For this review, take the finished solid that the model builds, in its own axes (mm). Coordinates: 2 decimals unless noted, no trailing zeros. Order: outer loops, then holes, each group sorted by start corner. A loop starts at its lowest first (then second) coordinate and runs counter-clockwise, first axis right, second up. Notation, with made-up numbers: (57, 3.25) -> (107, 3.25) arc R24 ccw to (107, 42.25) -> close; hole circle Ø7 at (62.25, 26). An arc over 180 degrees is marked (long way). Write item = value, one per line. Start each with the question number.
1) Consider section C-C on x = 88.9. Give the boundary of the cut face in (y, z).
2) Consider section B-B on z = -60.5. Give the boundary of the cut face in (x, y), and give its area (3 significant figures).
3) Consider section A-A on x = 50.8. Give the boundary of the cut face in (y, z), and give its area (3 significant figures).
4) Wall thickness on probe 1 along Z at (x, y) = (12.7, 3.75); probe 2 along X at (y, z) = (1.75, -31); probe 3 along X at (y, z) = (5, -19.05): over which ranges is each line inside the solid? List them lowest first. Write a range as [from, to].
5) Insertion check: pin 1 Ø6 at (x, z) = (50.8, -31.115) entering from -Y. The pin has a flat end and moves straight along its axis. Give the tip position at first contact, or say it passes through.
6) Consider section D-D on y = 4.5. State how many separate pieces and enclosed holes the cut face has, and give its area (3 significant figures).
7) Draft analysis for pull direction X (two halves, no side actions). For faces 1 (the face through (10.46, 3.13, -19.76)), 2 (the face through (101.6, 3, -35)), 3 (the face through (50, 3, -71.12)), 4 (the face through (0, 3, -35)), state which applies: +X half, -X half, draft (parallel to the pull), parting line (faces both ways), or undercut.
from build123d import *

# Parameters (mm, degrees)
SKETCH1_W                       = 101.6
SKETCH1_H                       = 71.12
BASE_DEPTH                      = 6.35
WOODSCREW_CLEARANCE_HOLES_D     = 4.699
WOODSCREW_CLEARANCE_HOLES_DEPTH = 6.35
WOODSCREW_CLEARANCE_HOLES_TIP   = 1.411722024
SHAFT_CLEARANCE_HOLE_D          = 10.2616
SHAFT_CLEARANCE_HOLE_DEPTH      = 6.35
SHAFT_CLEARANCE_HOLE_TIP        = 3.082895664
M5X0_8_TAPPED_HOLE1_D           = 4.2


with BuildPart() as part:
    # Sketch1 → base (new body)
    with BuildSketch(Plane(origin=(0, 0, 0), x_dir=(1, 0, 0), z_dir=(0, 1, 0))):
        with Locations((50.8, 35.56)):
            Rectangle(SKETCH1_W, SKETCH1_H)
    extrude(amount=BASE_DEPTH)

    # woodscrew clearance holes
    with Locations(Plane(origin=(0, 6.35, 0), x_dir=(1, 0, 0), z_dir=(0, 1, 0))):
        with Locations((12.7, 61.595), (88.9, 61.595), (88.9, 19.05), (12.7, 19.05)):
            Hole(WOODSCREW_CLEARANCE_HOLES_D / 2, depth=WOODSCREW_CLEARANCE_HOLES_DEPTH)
            with Locations((0, 0, -(WOODSCREW_CLEARANCE_HOLES_DEPTH + WOODSCREW_CLEARANCE_HOLES_TIP / 2))):  # 118° drill point
                Cone(0, WOODSCREW_CLEARANCE_HOLES_D / 2, WOODSCREW_CLEARANCE_HOLES_TIP, mode=Mode.SUBTRACT)

    # shaft clearance hole
    with Locations(Plane(origin=(0, 6.35, 0), x_dir=(1, 0, 0), z_dir=(0, 1, 0))):
        with Locations((50.8, 31.115)):
            Hole(SHAFT_CLEARANCE_HOLE_D / 2, depth=SHAFT_CLEARANCE_HOLE_DEPTH)
            with Locations((0, 0, -(SHAFT_CLEARANCE_HOLE_DEPTH + SHAFT_CLEARANCE_HOLE_TIP / 2))):  # 118° drill point
                Cone(0, SHAFT_CLEARANCE_HOLE_D / 2, SHAFT_CLEARANCE_HOLE_TIP, mode=Mode.SUBTRACT)

    # M5x0.8 Tapped Hole1 (through all)
    with Locations(Plane(origin=(0, 6.35, 0), x_dir=(1, 0, 0), z_dir=(0, 1, 0))):
        with Locations((32.258, 31.115), (69.342, 31.115)):
            Hole(M5X0_8_TAPPED_HOLE1_D / 2)


solid = part.part
Answer sheet:
q1.outline = (0, -71.12) -> (6.35, -71.12) -> (6.35, -63.94) -> (0, -63.94) -> close; (0, -59.25) -> (6.35, -59.25) -> (6.35, -21.4) -> (0, -21.4) -> close; (0, -16.7) -> (6.35, -16.7) -> (6.35, 0) -> (0, 0) -> close
q2.outline = (0, 0) -> (10.62, 0) -> (10.62, 6.35) -> (0, 6.35) -> close; (14.78, 0) -> (86.82, 0) -> (86.82, 6.35) -> (14.78, 6.35) -> close; (90.98, 0) -> (101.6, 0) -> (101.6, 6.35) -> (90.98, 6.35) -> close
q2.area = 592 mm2
q3.outline = (0, -71.12) -> (6.35, -71.12) -> (6.35, -36.25) -> (0, -36.25) -> close; (0, -25.98) -> (6.35, -25.98) -> (6.35, 0) -> (0, 0) -> close
q3.area = 386 mm2
q4.probe_1 = [-71.12, -63.94], [-59.25, -21.4], [-16.7, 0]
q4.probe_2 = [0, 30.16], [34.35, 45.67], [55.93, 67.25], [71.44, 101.6]
q4.probe_3 = [0, 10.35], [15.05, 86.55], [91.25, 101.6]
q5.pin_1 = through
q6.separate_pieces = 1
q6.enclosed_holes = 7
q6.area = 7,050 mm2
q7.face_1 = undercut
q7.face_2 = +X half
q7.face_3 = draft
q7.face_4 = -X half
